```python
from build123d import *

# Parameters (mm, degrees)
SKETCH_1_W          = 105
SKETCH_1_H          = 20
EXTRUDE_1_DEPTH     = 2
FILLET_1_R          = 3
SKETCH_2_R          = 2
SKETCH_2_R_2        = 1.6
CUT_EXTRUDE_1_DEPTH = 3


with BuildPart() as part:
    # 草图1 → 凸台-拉伸1 (new body)
    with BuildSketch(Plane.XY):
        Rectangle(SKETCH_1_W, SKETCH_1_H)
    extrude(amount=EXTRUDE_1_DEPTH)

    # 圆角1
    fillet_1_edges = [part.edges().sort_by_distance(p)[0] for p in [
        (52.5, -10, 1),
        (-52.5, -10, 1),
        (-52.5, 10, 1),
        (52.5, 10, 1),
    ]]
    fillet(fillet_1_edges, radius=FILLET_1_R)

    # 草图2 → 切除-拉伸1 (cut)
    with BuildSketch(Plane.XY.offset(2)):
        with Locations((-32.7, 5)):
            Circle(SKETCH_2_R)
        with Locations((-17.733222632, 5.997785158)):
            Circle(SKETCH_2_R)
        with Locations((17.7, 5)):
            Circle(SKETCH_2_R)
        with Locations((32.7, 5)):
            Circle(SKETCH_2_R)
        with Locations((42.5, -4.815743551)):
            Circle(SKETCH_2_R_2)
        with Locations((-42.5, -4.815743551)):
            Circle(SKETCH_2_R_2)
        with BuildLine():
            Line((-28.423476114, 2), (28.423476114, 2))
            ThreePointArc((28.423476114, 2), (30.544796458, 1.121320344), (31.423476114, -1))
            Line((31.423476114, -1), (31.423476114, -2))
            ThreePointArc((31.423476114, -2), (30.544796458, -4.121320344), (28.423476114, -5))
            Line((28.423476114, -5), (-28.423476114, -5))
            ThreePointArc((-28.423476114, -5), (-30.544796458, -4.121320344), (-31.423476114, -2))
            Line((-31.423476114, -2), (-31.423476114, -1))
            ThreePointArc((-31.423476114, -1), (-30.544796458, 1.121320344), (-28.423476114, 2))
        make_face()
    extrude(amount=-CUT_EXTRUDE_1_DEPTH, mode=Mode.SUBTRACT)


solid = part.part
```
The listing builds one solid part. Answer for the finished solid, in the listing's coordinates (mm). A direction names the side the tool comes from. Coordinates: 2 decimals unless noted, no trailing zeros. Write each loop counter-clockwise with the first axis right and the second up, starting at its lowest first coordinate (ties: lowest second). Pieces come first, ordered by that corner, then holes. Notation, with made-up numbers: (-40, -33.5) - (0, -33.5) arc R9 cw to (0, -29.5) - close; hole circle Ø1 at (-5.75, -7.75). An arc over 180 degrees is marked (long way). Return JSON: item names as keys, results as strings. Group by question number.
Q1. For a pull along X with two mould halves and no side action, classify faces 3 (the flat face through (-0.7, 2.4, 2)), 4 (the cylindrical face through (34.608, 5.601, 1.014)), 5 (the cylindrical face through (-51.64, -9.1, 1.01)) as +X half, -X half, draft (parallel to the pull), parting line (faces both ways), or undercut.
Q2. The part is cut by section C-C on x = 17.7. Write down the section's boundary in (y, z), and give its area (3 significant figures).
Q3. The part is cut by section D-D on z = 0.5. Write down the section's boundary in (x, y), and give its area (3 significant figures).
Q4. Which of the six approach directions +Z, -Z, +X, -X, +Y, -Y give full straight-line access (tool end or side, diameter ignored) to faces 1 (the cylindrical face through (51.64, 9.1, 1.01)), 2 (the flat face through (0, -5, 1))?
Q5. The part is cut by section B-B on y = 5. Write down the section's boundary in (x, z).
Q6. The part is cut by section A-A on x = -3.5. Write down the section's boundary in (y, z), and give its area (3 significant figures).
Q7. A flat-ended cylindrical pin translates along its axis: pin 1 Ø3.5 at (x, y) = (-32.7, 5) entering from -Z. Find the tip coordinate at first contact, or state that the pin passes through.
Q8. Find the intervals of material crossed by line 1 along Y through (x, z) = (17.7, 0.7); line 2 along Y through (x, z) = (-1, 0.15); line 3 along Y through (x, z) = (-32.5, 1.8), in increasing order. Write a range as [from, to].
Evaluation:
{
 "1": {"face 3": "draft", "face 4": "undercut", "face 5": "-X half"},
 "2": {"outline": "(-10, 0) - (-5, 0) - (-5, 2) - (-10, 2) - close; (2, 0) - (3, 0) - (3, 2) - (2, 2) - close; (7, 0) - (10, 0) - (10, 2) - (7, 2) - close", "area": "18.0 mm2"},
 "3": {"outline": "(-52.5, -7) arc R3 ccw to (-49.5, -10) - (49.5, -10) arc R3 ccw to (52.5, -7) - (52.5, 7) arc R3 ccw to (49.5, 10) - (-49.5, 10) arc R3 ccw to (-52.5, 7) - close; hole circle Ø3.2 at (-42.5, -4.82); hole circle Ø4 at (-32.7, 5); hole (-31.42, -2) arc R3 ccw to (-28.42, -5) - (28.42, -5) arc R3 ccw to (31.42, -2) - (31.42, -1) arc R3 ccw to (28.42, 2) - (-28.42, 2) arc R3 ccw to (-31.42, -1) - close; hole circle Ø4 at (-17.73, 6); hole circle Ø4 at (17.7, 5); hole circle Ø4 at (32.7, 5); hole circle Ø3.2 at (42.5, -4.82)", "area": "1,590 mm2"},
 "4": {"face 1": "+Z, -Z, +X, +Y", "face 2": "+Z, -Z"},
 "5": {"outline": "(-52.5, 0) - (-34.7, 0) - (-34.7, 2) - (-52.5, 2) - close; (-30.7, 0) - (-19.47, 0) - (-19.47, 2) - (-30.7, 2) - close; (-16, 0) - (15.7, 0) - (15.7, 2) - (-16, 2) - close; (19.7, 0) - (30.7, 0) - (30.7, 2) - (19.7, 2) - close; (34.7, 0) - (52.5, 0) - (52.5, 2) - (34.7, 2) - close"},
 "6": {"outline": "(-10, 0) - (-5, 0) - (-5, 2) - (-10, 2) - close; (2, 0) - (10, 0) - (10, 2) - (2, 2) - close", "area": "26.0 mm2"},
 "7": {"pin 1": "passes through"},
 "8": {"line 1": "y = [-10, -5], [2, 3], [7, 10]", "line 2": "y = [-10, -5], [2, 10]", "line 3": "y = [-10, 3.01], [6.99, 10]"}
}
